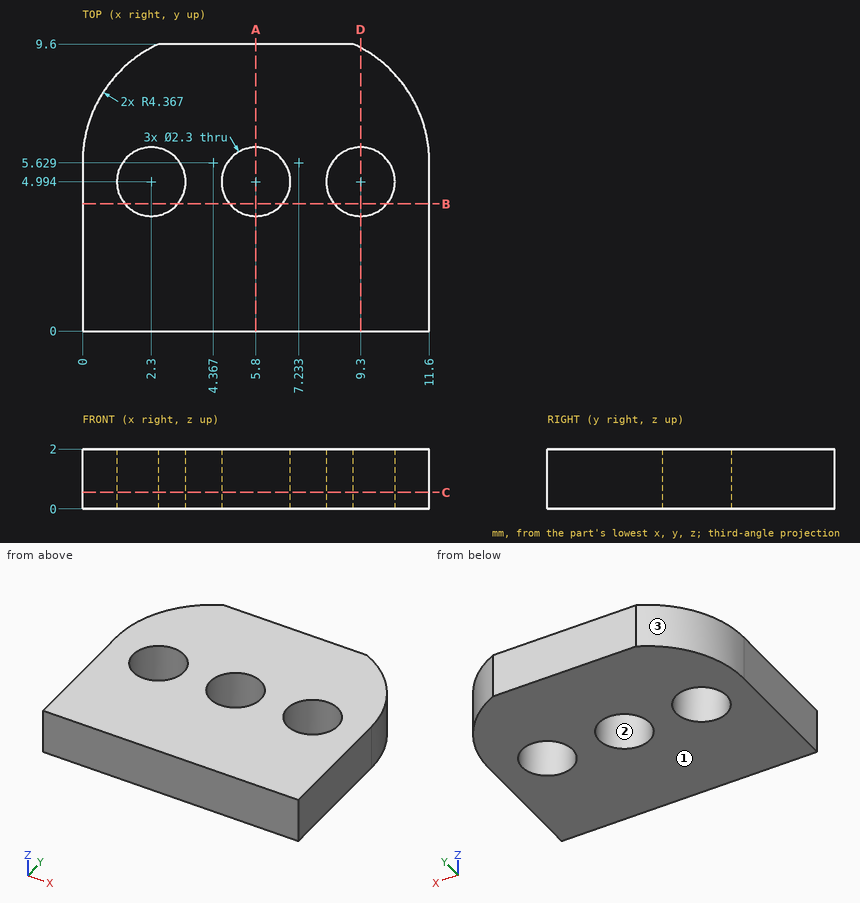
Check sheet for the drawn part. Datum: minimum x, y, z corner. Units: mm. Round coordinates to 2 decimals unless told otherwise and drop trailing zeros. Loops run counter-clockwise (first coordinate to the right, second up) from the corner with the lowest first, then second, coordinate; pieces in that order, holes last.
Item 1: Cross-section at C-C on z = 0.55. Record the boundary of the cut face in (x, y), then the cut area to 3 significant figures.
Item 2: Cross-section at D-D on x = 9.3. Record the boundary of the cut face in (y, z).
Item 3: Thickness scan on line 1 (X direction, y = 5, z = 0.95); line 2 (Y direction, x = 5.8, z = 0.6); line 3 (X direction, y = 4.5, z = 1.7). Record the ranges inside material, lowest first.
Item 4: Gauge pin test, flat end, axial feed: pin 1 (1.4 mm diameter, centred on x = 9.3, y = 4.99, fed in from -Z) (1 decimal). Record the tip position at first contact, or that the pin passes through.
Item 5: Cross-section at A-A on x = 5.8. Record the boundary of the cut face in (y, z), then the cut area to 3 significant figures.
Item 6: Cross-section at B-B on y = 4.25. Record the boundary of the cut face in (x, z), then the cut area to 3 significant figures.
Item 7: Mould release check, pull along X, two halves, no side actions. Record for the marked faces 1, 2 and 3: pulls with the +X half, pulls with the -X half, needs draft (parallel to the pull), parting line crosses it, or undercut.
Answer sheet:
1. outline: (0, 0) - (11.6, 0) - (11.6, 5.63) arc R4.37 ccw to (9.05, 9.6) - (2.55, 9.6) arc R4.37 ccw to (0, 5.63) - close; hole circle Ø2.3 at (2.3, 4.99); hole circle Ø2.3 at (5.8, 4.99); hole circle Ø2.3 at (9.3, 4.99)
1. area: 93.2 mm2
2. outline: (0, 0) - (3.84, 0) - (3.84, 2) - (0, 2) - close; (6.14, 0) - (9.48, 0) - (9.48, 2) - (6.14, 2) - close
3. line 1: x = 0 to 1.15, 3.45 to 4.65, 6.95 to 8.15, 10.45 to 11.6
3. line 2: y = 0 to 3.84, 6.14 to 9.6
3. line 3: x = 0 to 1.26, 3.34 to 4.76, 6.84 to 8.26, 10.34 to 11.6
4. pin 1: passes through
5. outline: (0, 0) - (3.84, 0) - (3.84, 2) - (0, 2) - close; (6.14, 0) - (9.6, 0) - (9.6, 2) - (6.14, 2) - close
5. area: 14.6 mm2
6. outline: (0, 0) - (1.42, 0) - (1.42, 2) - (0, 2) - close; (3.18, 0) - (4.92, 0) - (4.92, 2) - (3.18, 2) - close; (6.68, 0) - (8.42, 0) - (8.42, 2) - (6.68, 2) - close; (10.18, 0) - (11.6, 0) - (11.6, 2) - (10.18, 2) - close
6. area: 12.7 mm2
7. face 1: needs draft
7. face 2: undercut
7. face 3: pulls with the -X half
